from build123d import *

# Parameters (mm, degrees)
BOSS_EXTRUDE1_DEPTH = 15
SHELL1_T            = 3
SKETCH3_W           = 9
SKETCH3_H           = 11
CUT_EXTRUDE1_DEPTH  = 3
SKETCH4_R           = 2.5
CUT_EXTRUDE2_DEPTH  = 3
FILLET1_R           = 2
SKETCH5_R           = 3
BOSS_EXTRUDE2_DEPTH = 3.4
SKETCH6_R           = 1.9
BOSS_EXTRUDE3_DEPTH = 1.2


with BuildPart() as part:
    # Sketch1 → Boss-Extrude1 (new body)
    with BuildSketch(Plane(origin=(0, 0, 0), x_dir=(1, 0, 0), z_dir=(0, 1, 0))):
        Polygon((0, 0), (88, 0), (88, -41), (71.5, -41), (71.5, -111), (16.5, -111), (16.5, -41), (0, -41), align=None)
    extrude(amount=BOSS_EXTRUDE1_DEPTH)

    # Shell1
    shell1_openings = [part.faces().sort_by_distance(p)[0] for p in [
        (44, 15, 49.150442478),
    ]]
    offset(amount=SHELL1_T, openings=shell1_openings, kind=Kind.INTERSECTION)

    # Sketch3 → Cut-Extrude1 (cut)
    with BuildSketch(Plane(origin=(0, 0, -3), x_dir=(-1, 0, 0), z_dir=(0, 0, -1))):
        with Locations((-62, 9.5)):
            Rectangle(SKETCH3_W, SKETCH3_H)
    extrude(amount=-CUT_EXTRUDE1_DEPTH, mode=Mode.SUBTRACT)

    # Sketch4 → Cut-Extrude2 (cut)
    with BuildSketch(Plane.ZY.offset(3)):
        with Locations((26, 9)):
            Circle(SKETCH4_R)
    extrude(amount=-CUT_EXTRUDE2_DEPTH, mode=Mode.SUBTRACT)

    # Fillet1
    fillet1_edges = [part.edges().sort_by_distance(p)[0] for p in [
        (44, -3, 114),
        (13.5, -3, 79),
        (5.25, -3, 44),
        (-3, -3, 20.5),
        (-3, 6, -3),
        (91, 6, -3),
        (91, 6, 44),
        (74.5, 6, 44),
        (74.5, 6, 114),
        (13.5, 6, 114),
        (13.5, 6, 44),
        (-3, 6, 44),
        (44, -3, -3),
        (91, -3, 20.5),
        (82.75, -3, 44),
        (74.5, -3, 79),
    ]]
    fillet(fillet1_edges, radius=FILLET1_R)

    # Sketch5 → Boss-Extrude2 (add)
    with BuildSketch(Plane(origin=(0, 0, 0), x_dir=(1, 0, 0), z_dir=(0, 1, 0))):
        with Locations(Location((39.5, -80, 0), (0, 0, 90))):
            Circle(SKETCH5_R)
        with Locations(Location((79.5, -20, 0), (0, 0, 90))):
            Circle(SKETCH5_R)
    extrude(amount=BOSS_EXTRUDE2_DEPTH)

    # Sketch6 → Boss-Extrude3 (add)
    with BuildSketch(Plane(origin=(0, 3.4, 0), x_dir=(1, 0, 0), z_dir=(0, 1, 0))):
        with Locations(Location((39.5, -80, 0), (0, 0, 270))):
            Circle(SKETCH6_R)
        with Locations(Location((79.5, -20, 0), (0, 0, 270))):
            Circle(SKETCH6_R)
    extrude(amount=BOSS_EXTRUDE3_DEPTH)


solid = part.part
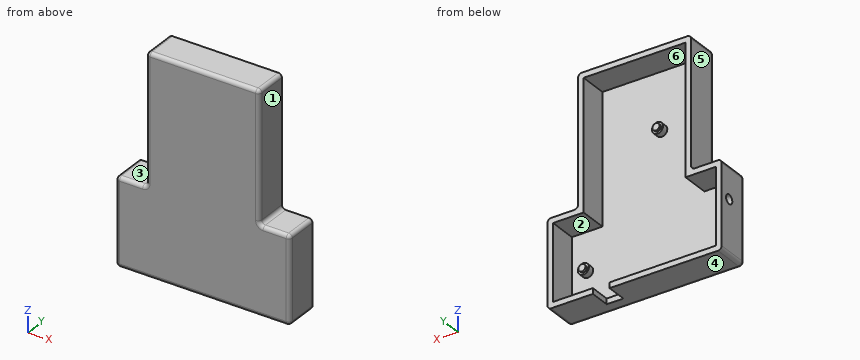
Can you work these out from the model? Positions are in its coordinate system, mm. Face numbers are marked on the shaded views. A direction names the side the tool comes from. Round coordinates to 2 decimals unless told otherwise and drop trailing zeros. Order: outer loops, then holes, each group sorted by start corner. A loop starts at its lowest first (then second) coordinate and runs counter-clockwise, first axis right, second up. Notation, with made-up numbers: (-15.75, -19.5) -> (15.25, -19.5) arc R23 ccw to (15.25, -11.5) -> close; hole circle Ø6 at (44.5, -24.5). An arc over 180 degrees is marked (long way). Write each question's results on one line, items separated by ' | '. Start each with the question number.
Item 1: Thinking about a two-plate mould opening in Z: for the marked faces 4, 5 and 6, which applies, +Z half, -Z half, draft (parallel to the pull), parting line (faces both ways), or undercut?
Item 2: If we section it at C-C, the plane y = 2: Write out the boundary of the cut face in (x, z).
Item 3: Please list where these lines run through material, in increasing order: L1, parallel to X at y = 11.5, z = 91.5; L2, parallel to Z at x = 22, y = 9.75; L3, parallel to X at y = 12.25, z = 30.
Item 4: If we section it at B-B, the plane z = 26: Write out the boundary of the cut face in (x, y), then the cut area to 3 significant figures.
Item 5: Which directions (+Z, -Z, +X, -X, +Y, -Y) give clear straight access to the entire face, cutting with the end or side of a thin tool? Please do the marked faces 1, 2 and 3.
Item 6: If we section it at D-D, the plane x = 7.5: Write out the boundary of the cut face in (y, z), then the cut area to 3 significant figures.
Item 7: Will these pins go through, and if not, where does the flat tip stop? pin 1 (5 mm diameter, centred on x = 79.5, z = 20.5, fed in from +Y); pin 2 (4.5 mm diameter, centred on y = 6.5, z = 83.5, fed in from +X); pin 3 (3.5 mm diameter, centred on x = 63, z = -2, fed in from +Y).
Results:
1) face 4: -Z half | face 5: draft | face 6: undercut
2) outline: (-3, -1) arc R2 ccw to (-1, -3) -> (89, -3) arc R2 ccw to (91, -1) -> (91, 42) arc R2 ccw to (89, 44) -> (76.5, 44) arc R2 cw to (74.5, 46) -> (74.5, 112) arc R2 ccw to (72.5, 114) -> (15.5, 114) arc R2 ccw to (13.5, 112) -> (13.5, 46) arc R2 cw to (11.5, 44) -> (-1, 44) arc R2 ccw to (-3, 42) -> close; circle Ø6 at (39.5, 80); circle Ø6 at (79.5, 20); hole (0, 0) -> (88, 0) -> (88, 41) -> (71.5, 41) -> (71.5, 111) -> (16.5, 111) -> (16.5, 41) -> (0, 41) -> close
3) L1: x = 13.5 to 16.5, 71.5 to 74.5 | L2: z = -3 to 0, 111 to 114 | L3: x = -3 to 0, 88 to 91
4) outline: (-3, -1) arc R2 ccw to (-1, -3) -> (89, -3) arc R2 ccw to (91, -1) -> (91, 15) -> (88, 15) -> (88, 0) -> (0, 0) -> (0, 6.5) -> (-3, 6.5) -> close; (-3, 11.5) -> (0, 11.5) -> (0, 15) -> (-3, 15) -> close | area: 355 mm2
5) face 1: +Z, +X, +Y, -Y | face 2: +Y | face 3: +Z, -X, +Y, -Y
6) outline: (-3, -1) arc R2 ccw to (-1, -3) -> (15, -3) -> (15, 0) -> (0, 0) -> (0, 41) -> (15, 41) -> (15, 44) -> (-1, 44) arc R2 ccw to (-3, 42) -> close | area: 229 mm2
7) pin 1: stops at y = 4.6 | pin 2: stops at x = 74.5 | pin 3: stops at y = 4
